Part model, mm, in its own coordinate system. Coordinates: 2 decimals unless noted, no trailing zeros. Write each loop counter-clockwise with the first axis right and the second up, starting at its lowest first coordinate (ties: lowest second). Pieces come first, ordered by that corner, then holes. Notation, with made-up numbers: (10.5, 24.5) -> (65.5, 24.5) arc R35 cw to (65.5, 63.5) -> close; hole circle Ø2 at (38.25, -16). An arc over 180 degrees is marked (long way). Write item = value, one per line.
from build123d import *

# Parameters (mm, degrees)
SKETCH_1_W             = 20
SKETCH_1_H             = 50
SM_BASE_FLANGE_1_DEPTH = 3
SKETCH_6_R             = 4
CUT_EXTRUDE_1_DEPTH    = 10
FILLET_1_R             = 4


# Sheet-metal steps are written as plain solids
with BuildPart() as part:
    # Sketch 1 → 基体-法兰1 (new body)
    with BuildSketch(Plane.XY):
        Rectangle(SKETCH_1_W, SKETCH_1_H)
    extrude(amount=-SM_BASE_FLANGE_1_DEPTH)

    # 草图6 → 切除-拉伸1 (cut)
    with BuildSketch(Plane.XY):
        with Locations((0, 17)):
            Circle(SKETCH_6_R)
        with Locations((0, -17)):
            Circle(SKETCH_6_R)
        Circle(SKETCH_6_R)
    extrude(amount=-CUT_EXTRUDE_1_DEPTH, mode=Mode.SUBTRACT)

    # 圆角1
    fillet_1_edges = [part.edges().sort_by_distance(p)[0] for p in [
        (10, -25, -1.5),
        (-10, -25, -1.5),
        (-10, 25, -1.5),
        (10, 25, -1.5),
    ]]
    fillet(fillet_1_edges, radius=FILLET_1_R)


solid = part.part
Q1. Saw through at B-B on y = 17. Give the cut face in (x, z), and give its area (3 significant figures).
Model answer:
outline = (-10, -3) -> (-4, -3) -> (-4, 0) -> (-10, 0) -> close; (4, -3) -> (10, -3) -> (10, 0) -> (4, 0) -> close
area = 36.0 mm²
Q2. Saw through at D-D on x = -3. Give the cut face in (y, z), and give its area (3 significant figures).
Model answer:
outline = (-25, -3) -> (-19.65, -3) -> (-19.65, 0) -> (-25, 0) -> close; (-14.35, -3) -> (-2.65, -3) -> (-2.65, 0) -> (-14.35, 0) -> close; (2.65, -3) -> (14.35, -3) -> (14.35, 0) -> (2.65, 0) -> close; (19.65, -3) -> (25, -3) -> (25, 0) -> (19.65, 0) -> close
area = 102 mm²
Q3. Saw through at A-A on x = 0. Give the cut face in (y, z).
Model answer:
outline = (-25, -3) -> (-21, -3) -> (-21, 0) -> (-25, 0) -> close; (-13, -3) -> (-4, -3) -> (-4, 0) -> (-13, 0) -> close; (4, -3) -> (13, -3) -> (13, 0) -> (4, 0) -> close; (21, -3) -> (25, -3) -> (25, 0) -> (21, 0) -> close
Q4. Saw through at C-C on z = -1.95. Give the cut face in (x, y).
Model answer:
outline = (-10, -21) arc R4 ccw to (-6, -25) -> (6, -25) arc R4 ccw to (10, -21) -> (10, 21) arc R4 ccw to (6, 25) -> (-6, 25) arc R4 ccw to (-10, 21) -> close; hole circle Ø8 at (0, -17); hole circle Ø8 at (0, 0); hole circle Ø8 at (0, 17)
Q5. Mould opens along X. For faces 1 (the face through (-0.521, -13.034, -1.479)), 2 (the face through (8.797, 23.859, -1.521)), 3 (the face through (0, -25, -1)) say: released by +X, released by -X, zero draft, split by the parting line, or undercut.
Model answer:
face_1 = undercut
face_2 = released by +X
face_3 = zero draft
Q6. Probe line 1 (Y direction, x = 0, z = -1.8); line 2 (X direction, y = -0.5, z = -2.7); line 3 (X direction, y = 18.5, z = -2.8). List the from-to ranges inside material, lowest first. Write a range as from..to.
Model answer:
line_1 = -25..-21, -13..-4, 4..13, 21..25
line_2 = -10..-3.97, 3.97..10
line_3 = -10..-3.71, 3.71..10
